Work out the finished part from the listing and answer in its coordinate system (mm). A direction names the side the tool comes from. Coordinates: 2 decimals unless noted, no trailing zeros. Order: outer loops, then holes, each group sorted by start corner. A loop starts at its lowest first (then second) coordinate and runs counter-clockwise, first axis right, second up. Notation, with made-up numbers: (79.5, 12.25) -> (105.5, 12.25) arc R29 cw to (105.5, 45.25) -> close; hole circle Ø7 at (84.25, 54). An arc over 180 degrees is marked (long way). Use one line per item in the form item = value.
from build123d import *

# Parameters (mm, degrees)
SKETCH1_W                                = 75
SKETCH1_H                                = 30
CBORE_FOR_M80_HEX_HEAD_BOLT1_D           = 85
CBORE_FOR_M80_HEX_HEAD_BOLT1_DEPTH       = 30
CBORE_FOR_M80_HEX_HEAD_BOLT1_CBORE_D     = 110
CBORE_FOR_M80_HEX_HEAD_BOLT1_CBORE_DEPTH = 22
HOLE1_D                                  = 8.376
HOLE1_DEPTH                              = 20
HOLE1_TIP                                = 2.516404272
M6_CLEARANCE_HOLE1_D                     = 6.647
M6_CLEARANCE_HOLE1_DEPTH                 = 12
M6_CLEARANCE_HOLE1_TIP                   = 1.996960267
CHAMFER1_SIZE                            = 1


with BuildPart() as part:
    # Sketch1 → Revolve1 (revolve)
    with BuildSketch(Plane(origin=(0, 0, 0), x_dir=(1, 0, 0), z_dir=(0, 1, 0))):
        with Locations((37.5, -15)):
            Rectangle(SKETCH1_W, SKETCH1_H)
    revolve(axis=Axis((0, 0, 0), (0, 0, 1)))

    # CBORE for M80 Hex Head Bolt1
    with Locations(Plane.XY.offset(30)):
        with Locations((0, 0)):
            CounterBoreHole(CBORE_FOR_M80_HEX_HEAD_BOLT1_D / 2, CBORE_FOR_M80_HEX_HEAD_BOLT1_CBORE_D / 2, CBORE_FOR_M80_HEX_HEAD_BOLT1_CBORE_DEPTH, depth=CBORE_FOR_M80_HEX_HEAD_BOLT1_DEPTH)

    # Hole1
    with Locations(Plane(origin=(0, 0, 0), x_dir=(-1, 0, 0), z_dir=(0, 0, -1))):
        with Locations((45.254833996, 45.254833996), (-45.254833996, 45.254833996), (-45.254833996, -45.254833996), (45.254833996, -45.254833996)):
            Hole(HOLE1_D / 2, depth=HOLE1_DEPTH)
            with Locations((0, 0, -(HOLE1_DEPTH + HOLE1_TIP / 2))):  # 118° drill point
                Cone(0, HOLE1_D / 2, HOLE1_TIP, mode=Mode.SUBTRACT)

    # M6 Clearance Hole1
    with Locations(Plane.XY.offset(30)):
        with Locations((0, 64), (0, -64), (64, 0), (-64, 0)):
            Hole(M6_CLEARANCE_HOLE1_D / 2, depth=M6_CLEARANCE_HOLE1_DEPTH)
            with Locations((0, 0, -(M6_CLEARANCE_HOLE1_DEPTH + M6_CLEARANCE_HOLE1_TIP / 2))):  # 118° drill point
                Cone(0, M6_CLEARANCE_HOLE1_D / 2, M6_CLEARANCE_HOLE1_TIP, mode=Mode.SUBTRACT)

    # Chamfer1
    chamfer1_edges = [part.edges().sort_by_distance(p)[0] for p in [
        (42.5, 0, 0),
        (-75, 0, 30),
        (-75, 0, 0),
    ]]
    chamfer(chamfer1_edges, length=CHAMFER1_SIZE)


solid = part.part
(1) Straight lines are drawn through the part: line 1 along Y through (x, z) = (0, 25.25); line 2 along X through (y, z) = (2, 20.75); line 3 along X through (y, z) = (-3, 23.5). For each, find the intervals that lie inside material, in ascending order.
Data:
line_1 = -75 to -67.32, -60.68 to -55, 55 to 60.68, 67.32 to 75
line_2 = -74.97 to -66.65, -61.35 to -54.96, 54.96 to 61.35, 66.65 to 74.97
line_3 = -74.94 to -65.43, -62.57 to -54.92, 54.92 to 62.57, 65.43 to 74.94
(2) Section A-A on z = 10.5 is taken. Write down the section's boundary in (x, y), plus the area to 3 significant figures.
Data:
outline = circle Ø150 at (0, 0); hole circle Ø110 at (0, 0); hole circle Ø8.38 at (-45.25, -45.25); hole circle Ø8.38 at (-45.25, 45.25); hole circle Ø8.38 at (45.25, -45.25); hole circle Ø8.38 at (45.25, 45.25)
area = 7,950 mm²
(3) Which of the six approach directions +Z, -Z, +X, -X, +Y, -Y give full straight-line access (tool end or side, diameter ignored) to faces 1 (the cylindrical face through (-1.79, 66.8, 23.92)), 2 (the cylindrical face through (-48.342, 48.085, 10.14)), 3 (the flat face through (-32, -32, 0))?
Data:
face_1 = +Z
face_2 = -Z
face_3 = -Z, +X, -X, +Y, -Y
(4) The mould has two halves that part along X. Classify faces 4 (the flat face through (55.2, 0.3, 30)), 5 (the conical face through (-44.68, -45.7, 22.08)): released by +X, released by -X, zero draft, split by the parting line, or undercut.
Data:
face_4 = zero draft
face_5 = undercut
(5) Each of these flat-tipped pins is pushed along its axis until it touches: P1, Ø10, axis at x = 11.5, z = 19.5, coming from the +Y side; P2, Ø12, axis at x = 11, z = 9, coming from the -Y side; P3, Ø2, axis at y = -23, z = 23.5, coming from the +X side; P4, Ø10, axis at x = -31.5, y = 17, coming from the -Z side. Where does it stop, or does it pass through?
Data:
P1 = 74.72
P2 = -74.83
P3 = 71.7
P4 = through
